Build history of the part. All positions in model axes, mm. A direction names the side the tool comes from. Coordinates: 2 decimals unless noted, no trailing zeros. Order: outer loops, then holes, each group sorted by start corner. A loop starts at its lowest first (then second) coordinate and runs counter-clockwise, first axis right, second up. Notation, with made-up numbers: M 20,51.5 L 77,51.5 A22 ccw 77,68.5 Z; hole C 83,-7 d6. An arc over 180 degrees is marked long. Use a Markdown table: item, result. Add a question column.
from build123d import *

# Parameters (mm, degrees)
EXTRUDE_1_DEPTH     = 10
EXTRUDE_2_DEPTH     = 3
SKETCH_3_R          = 2.1
CUT_EXTRUDE_1_DEPTH = 65.41273166075166
EXTRUDE_START       = -10
EXTRUDE_5_DEPTH     = 10
FILLET_1_R          = 30
FILLET_2_R          = 30


with BuildPart() as part:
    # 草圖1 → 填料-伸長1 (new body)
    with BuildSketch(Plane.XY):
        with BuildLine():
            Line((-39.999999999999964, -7.633e-14), (-37.499999999999964, -7.633e-14))
            ThreePointArc((-37.499999999999964, -7.633e-14), (-4.02e-14, 37.499999999999964), (37.5, 0))
            Line((37.5, 0), (40, 0))
            ThreePointArc((40, 0), (-4.288e-14, 39.999999999999964), (-39.999999999999964, -7.633e-14))
        make_face()
    extrude(amount=EXTRUDE_1_DEPTH)

    # 草圖2 → 填料-伸長2 (add)
    with BuildSketch(Plane(origin=(0, 0, 0), x_dir=(-1, 0, 0), z_dir=(0, 0, -1))):
        with BuildLine():
            Line((-39.99999999999998, -2.7932e-13), (-40, 50))
            Line((-40, 50), (40, 50))
            Line((40, 50), (39.999999999999964, -7.633e-14))
            ThreePointArc((39.999999999999964, -7.633e-14), (-1.1393e-13, 39.99999999999998), (-39.99999999999998, -2.7932e-13))
        make_face()
    extrude(amount=-EXTRUDE_2_DEPTH)

    # 草圖3 → 除料-伸長1 (cut, through all)
    with BuildSketch(Plane.XY.offset(3)):
        with Locations((-25, 42.5)):
            Circle(SKETCH_3_R)
        with Locations((25, 42.5)):
            Circle(SKETCH_3_R)
    extrude(amount=-CUT_EXTRUDE_1_DEPTH, mode=Mode.SUBTRACT)

    # 草圖4 → 填料-伸長5 (add)
    with BuildSketch(Plane(origin=(0, 0, 0), x_dir=(-1, 0, 0), z_dir=(0, 0, -1)).offset(EXTRUDE_START)):
        with BuildLine():
            Line((52.49999999999998, -12.500000000000076), (57.49999999999997, -12.500000000000076))
            ThreePointArc((57.49999999999997, -12.500000000000076), (52.37436867076461, -0.12563132923555287), (40.00000000000013, 4.999999999999924))
            Line((39.999999999999964, 4.999999999999924), (39.999999999999964, -7.633e-14))
            ThreePointArc((39.999999999999964, -7.461e-14), (48.83883476483181, -3.6611652351682356), (52.49999999999998, -12.500000000000078))
        make_face()
        with BuildLine():
            Line((39.999999999999964, -7.633e-14), (39.999999999999964, 4.999999999999924))
            ThreePointArc((40.00000000000013, 4.999999999999924), (39.84330526776641, 4.999298464821022), (39.686623098603214, 4.9971939155302305))
            ThreePointArc((39.68662309860321, 4.997193915530231), (39.92157890129177, 2.5035051483740323), (39.99999999999996, -2.809e-14))
        make_face()
    extrude_5 = extrude(amount=EXTRUDE_5_DEPTH)

    # 鏡射1: 填料-伸長5 across plane
    add(extrude_5.mirror(Plane(origin=(0, 0, 0), x_dir=(0, 0, 1), z_dir=(1, 0, 0))))

    # 圓角1
    fillet_1_edges = [part.edges().sort_by_distance(p)[0] for p in [
        (37.5, 4.27e-15, 5),
        (-37.49999999999997, -7.633e-14, 5),
    ]]
    fillet(fillet_1_edges, radius=FILLET_1_R)

    # 圓角2
    fillet_2_edges = [part.edges().sort_by_distance(p)[0] for p in [
        (-39.68662309860321, 4.997193915530232, 6.5),
        (39.68662309860321, 4.997193915530232, 6.5),
    ]]
    fillet(fillet_2_edges, radius=FILLET_2_R)


solid = part.part
(1) Slice it at D-D on x = 12.5. Give the cut face in (y, z), and give its area (3 significant figures).
(2) Slice it at B-B on x = -25. Give the cut face in (y, z).
(3) Slice it at C-C on y = 22.5. Give the cut face in (x, z), and give its area (3 significant figures).
(4) Drop flat-ended pins along their axis: P1, Ø5, axis at x = -25, y = 42.5, coming from the +Z side; P2, Ø2, axis at x = -0.5, z = 4, coming from the -Y side; P3, Ø1, axis at y = -6, z = 7, coming from the +X side; P4, Ø3.5, axis at x = 25, y = 42.5, coming from the -Z side. Give the stop position or say it passes through.
(5) Drill centre lines: line 1 along Z through (x, y) = (24.5, 37.5); line 2 along X through (y, z) = (-6.5, 5.5); line 3 along X through (y, z) = (32, 5). Where is each one in solid material? Low to high. Write a range as from..to.
(6) Slice it at A-A on y = 42.5. Give the cut face in (x, z).
(7) Which spindle directions (+Z, -Z, +X, -X, +Y, -Y) get a long thin tool onto all of the face, cutting with end or side? Do faces 5 (the cylindrical face through (50.97, -6.51, 5.07)), 6 (the cylindrical face through (0.644, 39.995, 6.451)), 7 (the flat face through (-40, 30, 1)). Say none if no direction does.
(8) Mould opens along X. For faces 1 (the cylindrical face through (-55.237, -3.892, 5.07)), 2 (the cylindrical face through (-50.97, -6.51, 5.07)), 3 (the cylindrical face through (25.969, 40.637, 1.521)), 4 (the flat face through (40, 30, 1)) say: released by +X, released by -X, zero draft, split by the parting line, or undercut.
Solutions:
| question | item | result |
|---|---|---|
| 1 | outline | M 35.36,0 L 50,0 L 50,3 L 38,3 L 38,10 L 35.36,10 Z |
| 1 | area | 62.4 mm² |
| 2 | outline | M 27.95,0 L 40.4,0 L 40.4,3 L 31.22,3 L 31.22,10 L 27.95,10 Z; M 44.6,0 L 50,0 L 50,3 L 44.6,3 Z |
| 3 | outline | M -40,0 L -30,0 L -30,10 L -33.07,10 L -33.07,3 L -40,3 Z; M 30,0 L 40,0 L 40,3 L 33.07,3 L 33.07,10 L 30,10 Z |
| 3 | area | 103 mm² |
| 4 | P1 | z = 3 |
| 4 | P2 | y = 37.47 |
| 4 | P3 | x = 56.44 |
| 4 | P4 | through |
| 5 | line 1 | 0..3 |
| 5 | line 2 | -56.44..-50.97, 50.97..56.44 |
| 5 | line 3 | -24..-19.55, 19.55..24 |
| 6 | outline | M -40,0 L -27.1,0 L -27.1,3 L -40,3 Z; M -22.9,0 L 22.9,0 L 22.9,3 L -22.9,3 Z; M 27.1,0 L 40,0 L 40,3 L 27.1,3 Z |
| 7 | face 5 | +Z, -Z, -Y |
| 7 | face 6 | +Z, +Y |
| 7 | face 7 | +Z, -Z, -X, +Y |
| 8 | face 1 | released by -X |
| 8 | face 2 | undercut |
| 8 | face 3 | undercut |
| 8 | face 4 | released by +X |
